Verification items for the finished model (mm, model axes). Round coordinates to 2 decimals unless told otherwise and drop trailing zeros. Write each loop counter-clockwise with the first axis right and the second up, starting at its lowest first coordinate (ties: lowest second). Pieces come first, ordered by that corner, then holes. Notation, with made-up numbers: M -38.75,23 L -15.75,23 A14 ccw -15.75,44 Z; hole C 0,48 d8. An arc over 180 degrees is marked long. Answer in a Markdown table with one row per item. Add a question column.
1. Sectioned sample at A-A on z = 1.25. Record the cut outline in (x, y), plus the area to 3 significant figures.
2. Material ranges on probe 1 along Z at (x, y) = (131, -217.5); probe 2 along Y at (x, z) = (136, 3.75); probe 3 along Z at (x, y) = (149, -128), recorded low to high.
3. Go/stop test with flat-tipped pins: pin 1 Ø1 at (y, z) = (-164.5, -1.5) entering from +X; pin 2 Ø10 at (x, y) = (120.5, -71) entering from -Z; pin 3 Ø3 at (x, z) = (165.5, -0.5) entering from -Y. Record where each tip stops, or that it passes through.
```python
from build123d import *

# Parameters (mm, degrees)
F3_DEPTH = 254


# Not quite as in the source:
# - a feature of the source that left no trace in its solid (it failed there, or was rolled back) is left out


with BuildPart() as f3:
    # F2 (on face) → F3 (new body)
    with BuildSketch(Plane(origin=(0, 0, 0), x_dir=(-0.9390877837, -0.3436773698, 0), z_dir=(-0.3436773698, 0.9390877837, 0))):
        Polygon((-2.54, -2.54), (0, 0), (0, 4.0038675896), (-203.2, 4.0038675896), (-203.2, 0), (-200.66, -2.54), (-198.12, 0), (-195.58, -2.54), (-193.04, 0), (-190.5, -2.54), (-187.96, 0), (-185.42, -2.54), (-182.88, 0), (-180.34, -2.54), (-177.8, 0), (-175.26, -2.54), (-172.72, 0), (-170.18, -2.54), (-167.64, 0), (-165.1, -2.54), (-162.56, 0), (-160.02, -2.54), (-157.48, 0), (-154.94, -2.54), (-152.4, 0), (-149.86, -2.54), (-147.32, 0), (-144.78, -2.54), (-142.24, 0), (-139.7, -2.54), (-137.16, 0), (-134.62, -2.54), (-132.08, 0), (-129.54, -2.54), (-127, 0), (-124.46, -2.54), (-121.92, 0), (-119.38, -2.54), (-116.84, 0), (-114.3, -2.54), (-111.76, 0), (-109.22, -2.54), (-106.68, 0), (-104.14, -2.54), (-101.6, 0), (-99.06, -2.54), (-96.52, 0), (-93.98, -2.54), (-91.44, 0), (-88.9, -2.54), (-86.36, 0), (-83.82, -2.54), (-81.28, 0), (-78.74, -2.54), (-76.2, 0), (-73.66, -2.54), (-71.12, 0), (-68.58, -2.54), (-66.04, 0), (-63.5, -2.54), (-60.96, 0), (-58.42, -2.54), (-55.88, 0), (-53.34, -2.54), (-50.8, 0), (-48.26, -2.54), (-45.72, 0), (-43.18, -2.54), (-40.64, 0), (-38.1, -2.54), (-35.56, 0), (-33.02, -2.54), (-30.48, 0), (-27.94, -2.54), (-25.4, 0), (-22.86, -2.54), (-20.32, 0), (-17.78, -2.54), (-15.24, 0), (-12.7, -2.54), (-10.16, 0), (-7.62, -2.54), (-5.08, 0), align=None)
    extrude(amount=-F3_DEPTH)


solid = f3.part
```
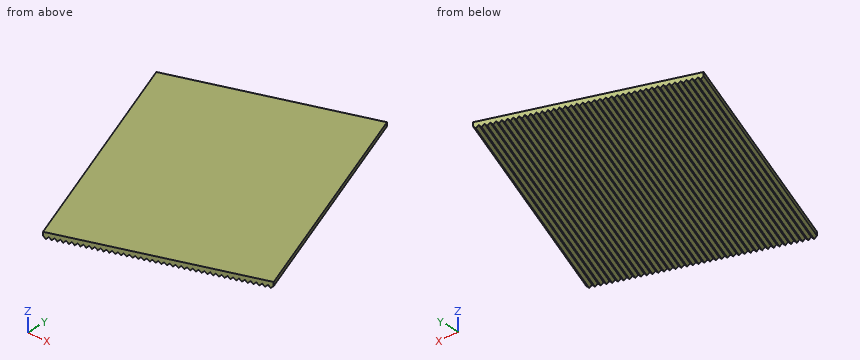
Geometry check:
| question | item | result |
|---|---|---|
| 1 | outline | M 0,0 L 87.29,-238.53 L 278.12,-168.69 L 190.82,69.84 Z |
| 1 | area | 51,600 mm2 |
| 2 | probe 1 | z = -2.53 to 4 |
| 2 | probe 2 | y = -220.7 to 49.77 |
| 2 | probe 3 | z = -0.59 to 4 |
| 3 | pin 1 | stops at x = 275.55 |
| 3 | pin 2 | stops at z = -2.54 |
| 3 | pin 3 | stops at y = -210.46 |
